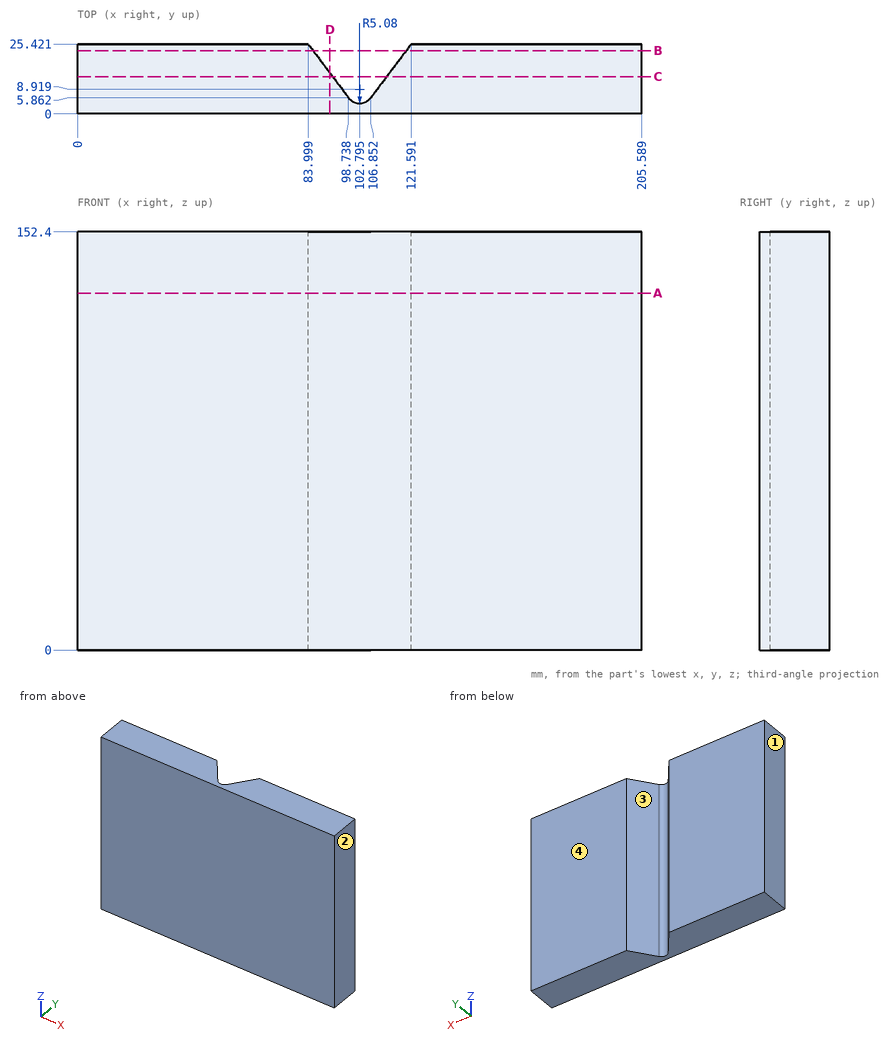
Check sheet for the drawn part. Datum: minimum x, y, z corner. Units: mm. Coordinates: 2 decimals unless noted, no trailing zeros. Loops run counter-clockwise (first coordinate to the right, second up) from the corner with the lowest first, then second, coordinate; pieces in that order, holes last. Notation, with made-up numbers: (77, 40.25) -> (118, 40.25) arc R17 cw to (118, 53.25) -> close; hole circle Ø5 at (60.5, -28.75). An arc over 180 degrees is marked (long way). Answer as a JSON object with one key per item and string values. Group by question number.
Item 1: Sectioned sample at C-C on y = 13.5. Record the boundary of the cut face in (x, z).
Item 2: Scan lines: probe 1 along X at (y, z) = (14.5, 64.5); probe 2 along X at (y, z) = (14.75, 43); probe 3 along Y at (x, z) = (112, 141) (1 decimal). Record each from-to range of solid material in increasing order.
Item 3: Sectioned sample at B-B on y = 23. Record the boundary of the cut face in (x, z).
Item 4: Sectioned sample at D-D on x = 92. Record the boundary of the cut face in (y, z), plus the area to 3 significant figures.
Item 5: Mould release check, pull along X, two halves, no side actions. Record for the marked faces 1, 2, 3 and 4: +X half, -X half, draft (parallel to the pull), parting line (faces both ways), or undercut.
Item 6: Sectioned sample at A-A on z = 130. Record the boundary of the cut face in (x, y) (1 decimal).
Evaluation:
{
 "1": {"outline": "(0, 0) -> (92.98, 0) -> (92.98, 152.4) -> (0, 152.4) -> close; (112.61, 0) -> (205.59, 0) -> (205.59, 152.4) -> (112.61, 152.4) -> close"},
 "2": {"probe 1": "x = 0 to 92.23, 113.36 to 205.59", "probe 2": "x = 0 to 92.04, 113.55 to 205.59", "probe 3": "y = 0 to 12.7"},
 "3": {"outline": "(0, 0) -> (85.82, 0) -> (85.82, 152.4) -> (0, 152.4) -> close; (119.77, 0) -> (205.59, 0) -> (205.59, 152.4) -> (119.77, 152.4) -> close"},
 "4": {"outline": "(0, 0) -> (14.8, 0) -> (14.8, 152.4) -> (0, 152.4) -> close", "area": "2,260 mm²"},
 "5": {"face 1": "-X half", "face 2": "+X half", "face 3": "undercut", "face 4": "draft"},
 "6": {"outline": "(0, 0) -> (205.6, 0) -> (205.6, 25.4) -> (121.6, 25.4) -> (106.9, 5.9) arc R5.1 cw to (98.7, 5.9) -> (84, 25.4) -> (0, 25.4) -> close"}
}
